Autodesk Inventor part; units mm, degrees
ref_plane "XZ Plane" through (0, 0, 0) normal (0, 1, 0) x (-1, 0, 0)
ref_plane "XY Plane" through (0, 0, 0) normal (0, 0, 1) x (1, 0, 0)
sketch "Sketch1" plane through (0, 0, 0) normal (0, 1, 0) x (-1, 0, 0)
  circle A0 centre (0, 0) radius 3.615
  circle A1 centre (0, 0) radius 5
  dimension "d0" = 7.23
  dimension "d1" = 10
extrude "Extrusion1" add sketch "Sketch1" along normal mid plane 40
ref_plane "Work Plane1" through (-5, 0, 0) normal (1, 0, 0) x (0, 1, 0)
sketch "Sketch2" plane through (-5, 0, 0) normal (1, 0, 0) x (0, 1, 0)
  circle A0 centre (0, 0) radius 3.615
  circle A1 centre (0, 0) radius 5
  dimension "d4" = 7.23
  dimension "d5" = 10
extrude "Extrusion2" add sketch "Sketch2" along normal blind 25 and the other way blind 15
sketch "Sketch3" plane through (20, 0, 0) normal (1, 0, 0) x (0, 0, -1)
  circle A0 centre (0, 0) radius 3.615
extrude "Extrusion3" cut sketch "Sketch3" against normal through all
sketch "Sketch4" plane through (0, -20, 0) normal (0, -1, 0) x (1, 0, 0)
  circle A0 centre (0, 0) radius 3.615
  dimension "d12" = 7.23
extrude "Extrusion4" cut sketch "Sketch4" against normal through all
properties part number "carrefour"
The listing builds one solid part. Answer for the finished solid, in the listing's coordinates (mm). A direction names the side the tool comes from. Give positions to 0.01 mm unless a question says otherwise; leave off trailing zeros. Order: outer loops, then holes, each group sorted by start corner. A loop starts at its lowest first (then second) coordinate and runs counter-clockwise, first axis right, second up. Notation, with made-up numbers: (-26.5, -30.75) -> (6.5, -30.75) arc R25 ccw to (6.5, -8.75) -> close; hole circle Ø11 at (-39, 19.5). An arc over 180 degrees is marked (long way). Write each question's results on one line, items separated by ' | '.
Q1. Each of these flat-tipped pins is pushed along its axis until it touches: P1, Ø2, axis at x = 13.5, y = -7.5, coming from the +Z side; P2, Ø2, axis at x = -14.5, z = -1.5, coming from the -Y side; P3, Ø6, axis at x = -5.5, z = 4, coming from the +Y side; P4, Ø4, axis at x = 15, z = -3, coming from the +Y side. Where does it stop, or does it pass through?
Checked values:
P1: passes through | P2: stops at y = -4.97 | P3: stops at y = 20 | P4: stops at y = 4.9
Q2. Which of the six approach directions +Z, -Z, +X, -X, +Y, -Y give full straight-line access (tool end or side, diameter ignored) to faces 1 (the face through (-12, 3, 4)), 2 (the face through (20, 3, 3)), 3 (the face through (-3, 20, 3)), 4 (the face through (-3, 12, -4)), 5 (the face through (-3, -12, 4))?
Checked values:
face 1: -X | face 2: +Z, -Z, +X, +Y, -Y | face 3: +Z, -Z, +X, -X, +Y | face 4: +Y | face 5: -Y
Q3. The part is cut by section D-D, the plane y = 8. Give the vertices of the cut face in (x, z) (3 decimals), and give its area (3 significant figures).
Checked values:
outline: circle Ø10 at (0, 0); hole circle Ø7.23 at (0, 0) | area: 37.5 mm^2
Q4. Determine the mould class of faces 6 (the face through (12, 3, -4)), 7 (the face through (-3, -20, 3)), 8 (the face through (12.082, 3.355, -1.345)) for opening direction Z: pulls with the +Z half, pulls with the -Z half, needs draft (parallel to the pull), parting line crosses it, or undercut.
Checked values:
face 6: parting line crosses it | face 7: needs draft | face 8: undercut
Q5. The part is cut by section B-B, the plane y = -2.5. Give the vertices of the cut face in (x, z) (3 decimals).
Checked values:
outline: (-20, -4.33) -> (-2.5, -4.33) arc R5 ccw to (2.5, -4.33) -> (20, -4.33) -> (20, -2.611) -> (2.5, -2.611) arc R3.615 cw to (-2.5, -2.611) -> (-20, -2.611) -> close; (-20, 2.611) -> (-2.5, 2.611) arc R3.615 cw to (2.5, 2.611) -> (20, 2.611) -> (20, 4.33) -> (2.5, 4.33) arc R5 ccw to (-2.5, 4.33) -> (-20, 4.33) -> close
Q6. Straight lines are drawn through the part: probe 1 along Y at (x, z) = (-15.5, 0) (3 decimals); probe 2 along Y at (x, z) = (-3.9, 0) (3 decimals). For each, find the intervals that lie inside material, in ascending order. Write a range as from..to.
Checked values:
probe 1: y = -5..-3.615, 3.615..5 | probe 2: y = -20..-3.615, 3.615..20
Q7. The part is cut by section A-A, the plane z = -0.5. Give the vertices of the cut face in (x, y), and give its area (3 significant figures).
Checked values:
outline: (-20, -4.97) -> (-4.97, -4.97) -> (-4.97, -20) -> (-3.58, -20) -> (-3.58, -3.58) -> (-20, -3.58) -> close; (-20, 3.58) -> (-3.58, 3.58) -> (-3.58, 20) -> (-4.97, 20) -> (-4.97, 4.97) -> (-20, 4.97) -> close; (3.58, -20) -> (4.97, -20) -> (4.97, -4.97) -> (20, -4.97) -> (20, -3.58) -> (3.58, -3.58) -> close; (3.58, 3.58) -> (20, 3.58) -> (20, 4.97) -> (4.97, 4.97) -> (4.97, 20) -> (3.58, 20) -> close | area: 175 mm^2
Q8. The part is cut by section C-C, the plane x = -4.5. Give the vertices of the cut face in (y, z) (3 decimals), and give its area (3 significant figures).
Checked values:
outline: (-20, -2.179) -> (-4.5, -2.179) arc R5 ccw to (4.5, -2.179) -> (20, -2.179) -> (20, 2.179) -> (4.5, 2.179) arc R5 ccw to (-4.5, 2.179) -> (-20, 2.179) -> close; hole circle Ø7.23 at (0, 0) | area: 170 mm^2
